Autodesk Inventor part; units mm, degrees
ref_plane "YZ Plane" through (0, 0, 0) normal (1, 0, 0) x (0, 1, 0)
ref_plane "XZ Plane" through (0, 0, 0) normal (0, 1, 0) x (-1, 0, 0)
ref_plane "XY Plane" through (0, 0, 0) normal (0, 0, 1) x (1, 0, 0)
sketch "Sketch1" plane through (0, 0, 0) normal (0, 0, 1) x (1, 0, 0)
  line L0 (0, 0) -> (144, 0)
  line L1 (144, 0) -> (144, 106)
  line L2 (144, 106) -> (0, 106)
  line L3 (0, 106) -> (0, 0)
  line L4 (21, 53) -> (46.5, 97.1673) construction
  line L5 (46.5, 97.1673) -> (97.5, 97.1673) construction
  line L6 (97.5, 97.1673) -> (123, 53) construction
  line L7 (123, 53) -> (97.5, 8.8327) construction
  line L8 (97.5, 8.8327) -> (46.5, 8.8327) construction
  line L9 (46.5, 8.8327) -> (21, 53) construction
  circle A0 centre (21, 53) radius 2.5
  circle A1 centre (46.5, 8.8327) radius 2.5
  circle A2 centre (97.5, 8.8327) radius 2.5
  circle A3 centre (123, 53) radius 2.5
  circle A4 centre (97.5, 97.1673) radius 2.5
  circle A5 centre (46.5, 97.1673) radius 2.5
  line L10 (9.5, 88) -> (9.5, 18) construction
  circle A6 centre (9.5, 88) radius 2.5
  circle A7 centre (9.5, 18) radius 2.5
  line L11 (134.5, 88) -> (134.5, 18) construction
  circle A8 centre (134.5, 88) radius 2.5
  circle A9 centre (134.5, 18) radius 2.5
  circle A10 centre (72, 53) radius 22.5
  point P0 (72, 106)
  point P1 (144, 53)
  point P2 (9.5, 53)
  point P3 (134.5, 53)
  dimension "d0" = 144
  dimension "d1" = 106
  dimension "d2" = 5
  dimension "d3" = 51
  dimension "d6" = 360
  dimension "d8" = 70
  dimension "d9" = 9.5
  dimension "d10" = 5
  dimension "d11" = 5
  dimension "d12" = 9.5
  dimension "d13" = 5
  dimension "d14" = 5
  dimension "d15" = 45
extrude "Extrusion1" add sketch "Sketch1" along normal blind 20
sketch "Sketch2" plane through (0, 0, 20) normal (0, 0, 1) x (1, 0, 0)
  circle A0 centre (46.5, 97.1673) radius 2.5 construction
  circle A1 centre (46.5, 97.1673) radius 6.5
  circle A2 centre (72, 53) radius 22.5 construction
  circle A3 centre (9.5, 88) radius 2.5 construction
  circle A4 centre (9.5, 18) radius 2.5 construction
  circle A5 centre (134.5, 88) radius 2.5 construction
  circle A6 centre (134.5, 18) radius 2.5 construction
  circle A7 centre (9.5, 88) radius 6.5
  circle A8 centre (9.5, 18) radius 6.5
  circle A9 centre (134.5, 18) radius 6.5
  circle A10 centre (134.5, 88) radius 6.5
  circle A11 centre (21, 53) radius 6.5
  circle A12 centre (46.5, 8.8327) radius 6.5
  circle A13 centre (97.5, 8.8327) radius 6.5
  circle A14 centre (123, 53) radius 6.5
  circle A15 centre (97.5, 97.1673) radius 6.5
  point P0 (0, 0)
  dimension "d18" = 13
  dimension "d19" = 13
  dimension "d20" = 13
  dimension "d21" = 13
  dimension "d22" = 13
  dimension "d25" = 360
extrude "Extrusion2" cut sketch "Sketch2" against normal blind 5 contours A7 | A8 | A9 | A10
properties part number "GA08" material "ABS Plastic"
Design review of the part built by this model. Coordinates are the model's own, in mm. A direction names the side the tool comes from. Coordinates: 2 decimals unless noted, no trailing zeros. Order: outer loops, then holes, each group sorted by start corner. A loop starts at its lowest first (then second) coordinate and runs counter-clockwise, first axis right, second up.
1) Take a section at B-B, the plane y = 18. Give the boundary of the cut face in (x, z), and give its area (3 significant figures).
2) Take a section at A-A, the plane x = 21. Give the boundary of the cut face in (y, z), and give its area (3 significant figures).
3) Clearance check with a flat-ended pin moving along its axis: pin 1 (6.5 mm diameter, centred on x = 135, y = 85, fed in from +Z). State where the tip first meets the part, or that it passes through.
4) For faces 1 (the cylindrical face through (54.145, 66.691, 9.86)), 2 (the cylindrical face through (8.091, 81.655, 17.535)), list the 3-axis set-ups (+Z, -Z, +X, -X, +Y, -Y) from which the entire face can be reached by the end or side of a thin tool; tool diameter is ignored.
5) Wall thickness on line 1 along X through (y, z) = (88, 7); line 2 along Y through (x, z) = (9.5, 9.25); line 3 along Y through (x, z) = (9.5, 17.5): over which ranges is each line inside the solid? List them lowest first.
6) Take a section at D-D, the plane y = 53. Give the boundary of the cut face in (x, z), and give its area (3 significant figures).
7) Mouldability with a two-part tool opening along Y and no side actions: class faces 3 (the flat face through (73, 106, 10)), 4 (the flat face through (144, 52, 10)), 5 (the cylindrical face through (136.885, 17.249, 7.395)) as +Y half, -Y half, draft (parallel to the pull), parting line (faces both ways), or undercut.
8) Take a section at C-C, the plane x = 134.5. Give the boundary of the cut face in (y, z), and give its area (3 significant figures).
Returned:
1. outline: (0, 0) - (7, 0) - (7, 15) - (3, 15) - (3, 20) - (0, 20) - close; (12, 0) - (132, 0) - (132, 15) - (128, 15) - (128, 20) - (16, 20) - (16, 15) - (12, 15) - close; (137, 0) - (144, 0) - (144, 20) - (141, 20) - (141, 15) - (137, 15) - close
1. area: 2,600 mm2
2. outline: (0, 0) - (50.5, 0) - (50.5, 20) - (0, 20) - close; (55.5, 0) - (106, 0) - (106, 20) - (55.5, 20) - close
2. area: 2,020 mm2
3. pin 1: stops at z = 15
4. face 1: +Z, -Z
4. face 2: +Z
5. line 1: x = 0 to 7, 12 to 132, 137 to 144
5. line 2: y = 0 to 15.5, 20.5 to 85.5, 90.5 to 106
5. line 3: y = 0 to 11.5, 24.5 to 81.5, 94.5 to 106
6. outline: (0, 0) - (18.5, 0) - (18.5, 20) - (0, 20) - close; (23.5, 0) - (49.5, 0) - (49.5, 20) - (23.5, 20) - close; (94.5, 0) - (120.5, 0) - (120.5, 20) - (94.5, 20) - close; (125.5, 0) - (144, 0) - (144, 20) - (125.5, 20) - close
6. area: 1,780 mm2
7. face 3: +Y half
7. face 4: draft
7. face 5: undercut
8. outline: (0, 0) - (15.5, 0) - (15.5, 15) - (11.5, 15) - (11.5, 20) - (0, 20) - close; (20.5, 0) - (85.5, 0) - (85.5, 15) - (81.5, 15) - (81.5, 20) - (24.5, 20) - (24.5, 15) - (20.5, 15) - close; (90.5, 0) - (106, 0) - (106, 20) - (94.5, 20) - (94.5, 15) - (90.5, 15) - close
8. area: 1,840 mm2
